Here's how the part is built. I have some questions about the finished solid (model axes, mm). Face numbers are marked on the shaded views. A direction names the side the tool comes from. Give positions to 0.01 mm unless a question says otherwise; leave off trailing zeros. Loops run counter-clockwise (first coordinate to the right, second up) from the corner with the lowest first, then second, coordinate; pieces in that order, holes last. Notation, with made-up numbers: M 68.5,-18 L 77.5,-18 A4 ccw 77.5,-14 Z; hole C 21.25,-32 d1. An arc over 180 degrees is marked long. Answer as CSV lines item,"result". Start each with the question number.
Item 1: I want a section at B-B on x = 5. List the corners of the cut face in (y, z) for me.
Item 2: I want a section at D-D on y = 80. List the corners of the cut face in (x, z) for me.
Item 3: I want a section at A-A on y = 49.5. List the corners of the cut face in (x, z) for me, plus the area to 3 significant figures.
Item 4: I want a section at C-C on z = 59.5. List the corners of the cut face in (x, y) for me, plus the area to 3 significant figures.
Item 5: If I drill on line 1 along Z through (x, y) = (26, 52); line 2 along Y through (x, z) = (2, -44.5); line 3 along X through (y, z) = (0.55, 93), over which ranges is the centre line in solid material (lowest first)? Write a range as from..to.
Item 6: For the marked faces 1 and 2, which set-ups out of +Z, -Z, +X, -X, +Y, -Y let a thin tool reach every point of the face, with its end or its side?
Item 7: Will these pins go through, and if not, where does the flat tip stop? P1, Ø11, axis at x = 5, z = 93, coming from the -Y side; P2, Ø4, axis at x = -13.5, z = 59, coming from the -Y side; P3, Ø5.5, axis at y = 8.5, z = -97, coming from the -X side; P4, Ø15.5, axis at x = 5, z = -93, coming from the -Y side.
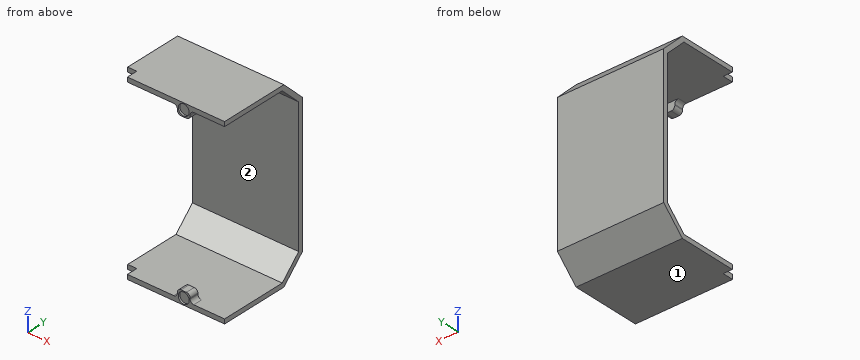
from build123d import *

# Parameters (mm, degrees)
SKETCH1_W           = 100
SKETCH1_H           = 5
BOSS_EXTRUDE1_DEPTH = 17
SKETCH6_W           = 10
SKETCH6_H           = 12
CUT_EXTRUDE1_DEPTH  = 234.428789998
SKETCH7_W           = 14
SKETCH7_H           = 14
BOSS_EXTRUDE2_DEPTH = 10
SKETCH8_R           = 6
CUT_EXTRUDE2_DEPTH  = 2
FILLET1_R           = 4
SKETCH9_W           = 14
SKETCH9_H           = 14
BOSS_EXTRUDE3_DEPTH = 10
SKETCH10_R          = 6
CUT_EXTRUDE3_DEPTH  = 2
FILLET2_R           = 4


with BuildPart() as part:
    # Sweep3: sweep along a path in Sketch2
    with BuildLine(Plane(origin=(0, 0, 0), x_dir=(0, 0, -1), z_dir=(1, 0, 0))) as sweep3_path:
        Line((-97.5, 0), (-97.5, 75))
        Line((-97.5, 75), (-75, 97.5))
        Line((-75, 97.5), (75, 97.5))
        Line((75, 97.5), (97.5, 75))
        Line((97.5, 75), (97.5, 0))
    # Sketch1 → Sweep3 (sweep)
    with BuildSketch(Plane(origin=(0, 0, 0), x_dir=(1, 0, 0), z_dir=(0, 1, 0))):
        with Locations((0, -97.5)):
            Rectangle(SKETCH1_W, SKETCH1_H)
    sweep(path=sweep3_path.line, transition=Transition.RIGHT)

    # Sketch5 → Boss-Extrude1 (add)
    with BuildSketch(Plane.ZY.offset(50)):
        Polygon((-100, 0), (-95, 0), (-95, 73.964466094), (-73.964466094, 95), (73.964466094, 95), (95, 73.964466094), (95, 0), (100, 0), (100, 76.035533906), (76.035533906, 100), (-76.035533906, 100), (-100, 76.035533906), align=None)
    extrude(amount=BOSS_EXTRUDE1_DEPTH)

    # Sketch6 → Cut-Extrude1 (cut, through all)
    with BuildSketch(Plane(origin=(0, 0, -100), x_dir=(-1, 0, 0), z_dir=(0, 0, -1))):
        with Locations((62, 6)):
            Rectangle(SKETCH6_W, SKETCH6_H)
    extrude(amount=-CUT_EXTRUDE1_DEPTH, mode=Mode.SUBTRACT)

    # Sketch7 → Boss-Extrude2 (add)
    with BuildSketch(Plane.XZ):
        with Locations((5, 93)):
            Rectangle(SKETCH7_W, SKETCH7_H)
    extrude(amount=-BOSS_EXTRUDE2_DEPTH)

    # Sketch8 → Cut-Extrude2 (cut)
    with BuildSketch(Plane.XZ):
        with Locations(Location((5, 93, 0), (0, 0, 270))):
            Circle(SKETCH8_R)
    extrude(amount=-CUT_EXTRUDE2_DEPTH, mode=Mode.SUBTRACT)

    # Fillet1
    fillet1_edges = [part.edges().sort_by_distance(p)[0] for p in [
        (12, 5, 95),
        (-2, 5, 95),
        (-2, 5, 86),
        (12, 5, 86),
    ]]
    fillet(fillet1_edges, radius=FILLET1_R)

    # Sketch9 → Boss-Extrude3 (add)
    with BuildSketch(Plane.XZ):
        with Locations((5, -93)):
            Rectangle(SKETCH9_W, SKETCH9_H)
    extrude(amount=-BOSS_EXTRUDE3_DEPTH)

    # Sketch10 → Cut-Extrude3 (cut)
    with BuildSketch(Plane.XZ):
        with Locations(Location((5, -93, 0), (0, 0, 270))):
            Circle(SKETCH10_R)
    extrude(amount=-CUT_EXTRUDE3_DEPTH, mode=Mode.SUBTRACT)

    # Fillet2
    fillet2_edges = [part.edges().sort_by_distance(p)[0] for p in [
        (12, 5, -86),
        (-2, 5, -95),
        (-2, 5, -86),
        (12, 5, -95),
    ]]
    fillet(fillet2_edges, radius=FILLET2_R)


solid = part.part
Result:
1,outline,"M 0,-100 L 76.04,-100 L 100,-76.04 L 100,76.04 L 76.04,100 L 0,100 L 0,99 L 2,99 L 2,87 L 0,87 L 0,86 L 10,86 L 10,95 L 73.96,95 L 95,73.96 L 95,-73.96 L 73.96,-95 L 10,-95 L 10,-86 L 0,-86 L 0,-87 L 2,-87 L 2,-99 L 0,-99 Z"
2,outline,"M -67,-96.04 L 50,-96.04 L 50,-88.96 L -67,-88.96 Z; M -67,88.96 L 50,88.96 L 50,96.04 L -67,96.04 Z"
3,outline,"M -67,-100 L 50,-100 L 50,-95 L -67,-95 Z; M -67,95 L 50,95 L 50,100 L -67,100 Z"
3,area,"1,170 mm^2"
4,outline,"M -67,95 L 50,95 L 50,100 L -67,100 Z"
4,area,"585 mm^2"
5,line 1,"-100..-95, 95..100"
5,line 2,"95..100"
5,line 3,"-2.54..-1, 11..12.54"
6,face 1,"-Z, +X, -X, +Y, -Y"
6,face 2,"+X, -X, -Y"
7,P1,"y = 2"
7,P2,"y = 95"
7,P3,"x = -57"
7,P4,"y = 0"
